from build123d import *

# Parameters (mm, degrees)
EXTRUDE_1_DEPTH     = 3
SKETCH_2_R          = 20
EXTRUDE_2_DEPTH     = 3
FILLET_1_R          = 10
SKETCH_3_R          = 2
SKETCH_3_R_2        = 5
CUT_EXTRUDE_1_DEPTH = 3


with BuildPart() as part:
    # 草图1 → 凸台-拉伸1 (new body)
    with BuildSketch(Plane.XY):
        with BuildLine():
            Line((0, 16), (100, 16))
            ThreePointArc((100, 16), (116, 0), (100, -16))
            Line((100, -16), (0, -16))
            ThreePointArc((0, -16), (-16, 0), (0, 16))
        make_face()
    extrude(amount=EXTRUDE_1_DEPTH)

    # 草图2 → 凸台-拉伸2 (add)
    with BuildSketch(Plane.XY.offset(3)):
        Circle(SKETCH_2_R)
    extrude(amount=-EXTRUDE_2_DEPTH)

    # 圆角1
    fillet_1_edges = [part.edges().sort_by_distance(p)[0] for p in [
        (12, -16, 1.5),
        (12, 16, 1.5),
    ]]
    fillet(fillet_1_edges, radius=FILLET_1_R)

    # 草图3 → 切除-拉伸1 (cut)
    with BuildSketch(Plane.XY.offset(3)):
        with Locations((0, 13)):
            Circle(SKETCH_3_R)
        with Locations((13, 0)):
            Circle(SKETCH_3_R)
        with Locations((0, -13)):
            Circle(SKETCH_3_R)
        with Locations((-13, 0)):
            Circle(SKETCH_3_R)
        Circle(SKETCH_3_R_2)
        with Locations((100, 0)):
            Circle(SKETCH_3_R_2)
    extrude(amount=-CUT_EXTRUDE_1_DEPTH, mode=Mode.SUBTRACT)


solid = part.part
Build history of the part. All positions in model axes, mm. A direction names the side the tool comes from. Coordinates: 2 decimals unless noted, no trailing zeros. Write each loop counter-clockwise with the first axis right and the second up, starting at its lowest first coordinate (ties: lowest second). Pieces come first, ordered by that corner, then holes.
(1) Cut at D-D on x = 101.5. List the corners of the cut face in (y, z), and give its area (3 significant figures).
(2) Cut at C-C on z = 1.65. List the corners of the cut face in (x, y).
(3) Mould opens along Y. For faces 4 (the cylindrical face through (116, 0, 1)), 5 (the cylindrical face through (0, 15, 2)), 6 (the flat face through (47, 0, 3)), 7 (the cylindrical face through (12.35, -16.35, 1.52)) say: pulls with the +Y half, pulls with the -Y half, needs draft (parallel to the pull), parting line crosses it, or undercut.
(4) Cut at A-A on y = 0. List the corners of the cut face in (x, z).
(5) Drill centre lines: line 1 (Y direction, x = 100, z = 1); line 2 (X direction, y = 4, z = 2.75); line 3 (Y direction, x = 61.5, z = 2.6). Where is each one in solid material? Low to high.
(6) 3-axis set-ups, long thin cutter, end or side, ignore diameter. For faces 1 (the flat face through (58, -16, 1)), 2 (the cylindrical face through (0, -11, 2)), 3 (the flat face through (57, 16, 1)): which of +Z, -Z, +X, -X, +Y, -Y reach the whole face in a straight line?
(7) Pin check, flat tips, straight feed: pin 1 Ø1.5 at (x, z) = (70, 1.5) entering from -Y; pin 2 Ø2.5 at (x, y) = (13, 0) entering from -Z; pin 3 Ø1.5 at (y, z) = (-1, 0.5) entering from +X; pin 4 Ø1 at (y, z) = (1, 1) entering from -X. Stop position of each tip, or through.
(8) Cut at B-B on x = 0. List the corners of the cut face in (y, z), and give its area (3 significant figures).
Working result:
1. outline: (-15.93, 0) - (-4.77, 0) - (-4.77, 3) - (-15.93, 3) - close; (4.77, 0) - (15.93, 0) - (15.93, 3) - (4.77, 3) - close
1. area: 67.0 mm2
2. outline: (9.98, -17.33) arc R10 cw to (14.97, -16) - (100, -16) arc R16 ccw to (100, 16) - (14.97, 16) arc R10 cw to (9.98, 17.33) arc R20 ccw (long way) to start; hole circle Ø4 at (-13, 0); hole circle Ø10 at (0, 0); hole circle Ø4 at (0, -13); hole circle Ø4 at (0, 13); hole circle Ø4 at (13, 0); hole circle Ø10 at (100, 0)
3. face 4: parting line crosses it
3. face 5: undercut
3. face 6: needs draft
3. face 7: pulls with the -Y half
4. outline: (-20, 0) - (-15, 0) - (-15, 3) - (-20, 3) - close; (-11, 0) - (-5, 0) - (-5, 3) - (-11, 3) - close; (5, 0) - (11, 0) - (11, 3) - (5, 3) - close; (15, 0) - (95, 0) - (95, 3) - (15, 3) - close; (105, 0) - (116, 0) - (116, 3) - (105, 3) - close
5. line 1: y = -16 to -5, 5 to 16
5. line 2: x = -19.6 to -3, 3 to 97, 103 to 115.49
5. line 3: y = -16 to 16
6. face 1: +Z, -Z, +X, -Y
6. face 2: +Z, -Z
6. face 3: +Z, -Z, +X, +Y
7. pin 1: stops at y = -16
7. pin 2: passes through
7. pin 3: stops at x = 116
7. pin 4: stops at x = -19.99
8. outline: (-20, 0) - (-15, 0) - (-15, 3) - (-20, 3) - close; (-11, 0) - (-5, 0) - (-5, 3) - (-11, 3) - close; (5, 0) - (11, 0) - (11, 3) - (5, 3) - close; (15, 0) - (20, 0) - (20, 3) - (15, 3) - close
8. area: 66.0 mm2
